```python
from build123d import *

# Parameters (mm, degrees)
SKETCH1_W           = 16.8
SKETCH1_H           = 16.8
SKETCH1_W_2         = 12.8
SKETCH1_H_2         = 12.8
BOSS_EXTRUDE1_DEPTH = 15
CUT_EXTRUDE1_DEPTH  = 17.8


with BuildPart() as part:
    # Sketch1 → Boss-Extrude1 (new body)
    with BuildSketch(Plane.XY):
        Rectangle(SKETCH1_W, SKETCH1_H)
        Rectangle(SKETCH1_W_2, SKETCH1_H_2, mode=Mode.SUBTRACT)
    extrude(amount=BOSS_EXTRUDE1_DEPTH)

    # Sketch2 → Cut-Extrude1 (cut, through all)
    with BuildSketch(Plane(origin=(8.4, 0, 0), x_dir=(0, 0, -1), z_dir=(1, 0, 0))):
        Polygon((-15, 6.4), (-2, -8.4), (-15, -8.4), align=None)
    extrude(amount=-CUT_EXTRUDE1_DEPTH, mode=Mode.SUBTRACT)


solid = part.part
```
Source: CAD feature listing. Evaluate the final solid. Frame: model axes, mm. A direction names the side the tool comes from. Give positions to 0.01 mm unless a question says otherwise; leave off trailing zeros. Order: outer loops, then holes, each group sorted by start corner. A loop starts at its lowest first (then second) coordinate and runs counter-clockwise, first axis right, second up.
(1) Section query B-B (y = 2.25). Return the cut outline in (x, z), plus the area to 3 significant figures.
(2) Contact query for a flat-ended pin moving along its axis: P1, Ø6, axis at x = 0, z = 12.5, coming from the -Y side. Output: stop coordinate, or through.
(3) Access query for faces 1 (the face through (8.4, 2, 6)), 2 (the face through (6.4, 1, 6)). Directions: +Z, -Z, +X, -X, +Y, -Y. A direction counts if a zero-diameter tool reaches every point of the face in a straight line with its end or side. Return the directions, or none.
(4) Material intervals for line 1 along Y through (x, z) = (4.75, 1); line 2 along Y through (x, z) = (5.25, 13), sorted ascending.
(5) Section query A-A (x = -2.5). Return the cut outline in (y, z).
(6) Pull-direction query (Y, two-part tool) for faces 3 (the face through (0, 6.4, 7)), 4 (the face through (-8, 0, 0)), 5 (the face through (0, 8.4, 7)); classes: +Y half, -Y half, draft (parallel to the pull), parting line (faces both ways), or undercut.
(7) Section query C-C (z = 5.5). Return the cut outline in (x, y), plus the area to 3 significant figures.
(8) Section query D-D (x = -7). Return the cut outline in (y, z).
Outcome:
1. outline: (-8.4, 0) - (-6.4, 0) - (-6.4, 11.35) - (-8.4, 11.35) - close; (6.4, 0) - (8.4, 0) - (8.4, 11.35) - (6.4, 11.35) - close
1. area: 45.4 mm2
2. P1: stops at y = 6.4
3. face 1: +Z, -Z, +X, +Y, -Y
3. face 2: +Z, -Z
4. line 1: y = -8.4 to -6.4, 6.4 to 8.4
4. line 2: y = 6.4 to 8.4
5. outline: (-8.4, 0) - (-6.4, 0) - (-6.4, 3.76) - (-8.4, 2) - close; (6.4, 0) - (8.4, 0) - (8.4, 15) - (6.4, 15) - close
6. face 3: undercut
6. face 4: draft
6. face 5: +Y half
7. outline: (-8.4, -4.42) - (-6.4, -4.42) - (-6.4, 6.4) - (6.4, 6.4) - (6.4, -4.42) - (8.4, -4.42) - (8.4, 8.4) - (-8.4, 8.4) - close
7. area: 76.9 mm2
8. outline: (-8.4, 0) - (8.4, 0) - (8.4, 15) - (6.4, 15) - (-8.4, 2) - close
